Can you work these out from the model? Positions are in its coordinate system, mm. Give positions to 0.01 mm unless a question says otherwise; leave off trailing zeros. Write each loop counter-clockwise with the first axis right and the second up, starting at its lowest first coordinate (ties: lowest second). Pieces come first, ordered by that corner, then holes. Notation, with made-up numbers: M 64,25 L 79,25 A30 cw 79,53 Z; hole C 64,32 d10. An arc over 180 degrees is marked long. Write each question's results on one line, items separated by ' | '.
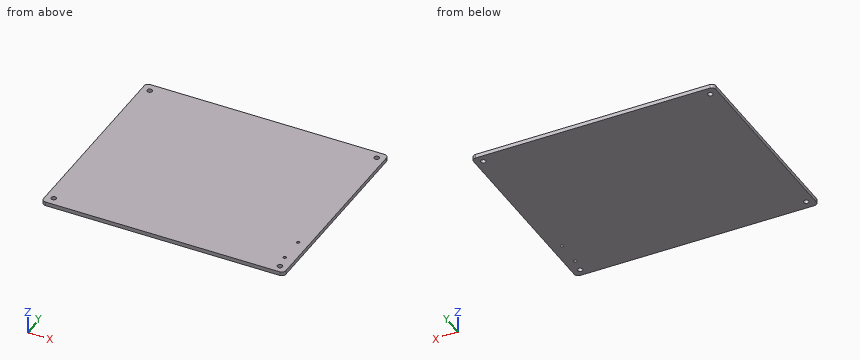
from build123d import *

# Parameters (mm, degrees)
SKETCH1_R           = 3.25
SKETCH1_R_2         = 1.9
BOSS_EXTRUDE1_DEPTH = 5


with BuildPart() as part:
    # Sketch1 → Boss-Extrude1 (new body)
    with BuildSketch(Plane.XY):
        with BuildLine():
            Line((-295, -10), (5, -10))
            ThreePointArc((5, -10), (8.535533906, -8.535533906), (10, -5))
            Line((10, -5), (10, 245))
            ThreePointArc((10, 245), (8.535533906, 248.535533906), (5, 250))
            Line((5, 250), (-295, 250))
            ThreePointArc((-295, 250), (-298.535533906, 248.535533906), (-300, 245))
            Line((-300, 245), (-300, -5))
            ThreePointArc((-300, -5), (-298.535533906, -8.535533906), (-295, -10))
        make_face()
        Circle(SKETCH1_R, mode=Mode.SUBTRACT)
        with Locations((0, 240)):
            Circle(SKETCH1_R, mode=Mode.SUBTRACT)
        with Locations((-290, 239)):
            Circle(SKETCH1_R, mode=Mode.SUBTRACT)
        with Locations((-290, 1)):
            Circle(SKETCH1_R, mode=Mode.SUBTRACT)
        with Locations((-3.100000029, 17.782619509)):
            Circle(SKETCH1_R_2, mode=Mode.SUBTRACT)
        with Locations((-3.100000029, 51.217380491)):
            Circle(SKETCH1_R_2, mode=Mode.SUBTRACT)
    extrude(amount=BOSS_EXTRUDE1_DEPTH)


solid = part.part
Item 1: If I drill on line 1 (Y direction, x = 0, z = 3.6); line 2 (X direction, y = 240, z = 3.75); line 3 (X direction, y = 239, z = 3.45), over which ranges is the centre line in solid material (lowest first)? Write a range as from..to.
Geometry says:
line 1: y = -10..-3.25, 3.25..236.75, 243.25..250 | line 2: x = -300..-293.09, -286.91..-3.25, 3.25..10 | line 3: x = -300..-293.25, -286.75..-3.09, 3.09..10
Item 2: I'm going to push a flat-ended pin straight in: pin 1 (10.5 mm diameter, centred on x = 0, y = 240, fed in from -Z). Where does the tip first touch, or does it pass through?
Geometry says:
pin 1: stops at z = 0
Item 3: I want a section at A-A, the plane x = -290. Please give me the cut outline in (y, z), and give its area (4 significant figures).
Geometry says:
outline: M -10,0 L -2.25,0 L -2.25,5 L -10,5 Z; M 4.25,0 L 235.75,0 L 235.75,5 L 4.25,5 Z; M 242.25,0 L 250,0 L 250,5 L 242.25,5 Z | area: 1,235 mm2
